Work out the finished part from the listing and answer in its coordinate system (mm). Round coordinates to 2 decimals unless told otherwise and drop trailing zeros. Loops run counter-clockwise (first coordinate to the right, second up) from the corner with the lowest first, then second, coordinate; pieces in that order, holes last.
Autodesk Inventor part; units mm, degrees
ref_plane "YZ Plane" through (0, 0, 0) normal (1, 0, 0) x (0, 1, 0)
ref_plane "XZ Plane" through (0, 0, 0) normal (0, 1, 0) x (-1, 0, 0)
ref_plane "XY Plane" through (0, 0, 0) normal (0, 0, 1) x (1, 0, 0)
sketch "Foam Scheme" plane through (0, 0, 0) normal (0, 1, 0) x (-1, 0, 0)
  line L0 (447, -94) -> (-447, -94)
  line L1 (-447, -94) -> (-447, 94)
  line L2 (-447, 94) -> (447, 94)
  line L3 (447, 94) -> (447, -94)
  circle A0 centre (425, -72) radius 9.5
  circle A1 centre (375, -72) radius 9.5
  circle A2 centre (325, -72) radius 9.5
  circle A3 centre (275, -72) radius 9.5
  circle A4 centre (225, -72) radius 9.5
  circle A5 centre (175, -72) radius 9.5
  circle A6 centre (125, -72) radius 9.5
  circle A7 centre (75, -72) radius 9.5
  circle A8 centre (25, -72) radius 9.5
  circle A9 centre (-25, -72) radius 9.5
  circle A10 centre (-75, -72) radius 9.5
  circle A11 centre (-125, -72) radius 9.5
  circle A12 centre (-175, -72) radius 9.5
  circle A13 centre (-225, -72) radius 9.5
  circle A14 centre (-275, -72) radius 9.5
  circle A15 centre (-325, -72) radius 9.5
  circle A16 centre (-375, -72) radius 9.5
  circle A17 centre (-425, -72) radius 9.5
  circle A18 centre (425, 72) radius 9.5
  circle A19 centre (375, 72) radius 9.5
  circle A20 centre (325, 72) radius 9.5
  circle A21 centre (275, 72) radius 9.5
  circle A22 centre (225, 72) radius 9.5
  circle A23 centre (175, 72) radius 9.5
  circle A24 centre (125, 72) radius 9.5
  circle A25 centre (75, 72) radius 9.5
  circle A26 centre (25, 72) radius 9.5
  circle A27 centre (-25, 72) radius 9.5
  circle A28 centre (-75, 72) radius 9.5
  circle A29 centre (-125, 72) radius 9.5
  circle A30 centre (-175, 72) radius 9.5
  circle A31 centre (-225, 72) radius 9.5
  circle A32 centre (-275, 72) radius 9.5
  circle A33 centre (-325, 72) radius 9.5
  circle A34 centre (-375, 72) radius 9.5
  circle A35 centre (-425, 72) radius 9.5
  point P0 (0, 0)
  dimension "d0" = 894
  dimension "d1" = 447
  dimension "d2" = 188
  dimension "d3" = 94
  dimension "d4" = 19
  dimension "d5" = 22
  dimension "d6" = 22
  dimension "d9" = 50
  dimension "d12" = 144
extrude "Foam Body" add sketch "Foam Scheme" along normal blind 1.5
properties part number "Foam NPS 6" material "Rubber, Silicone"
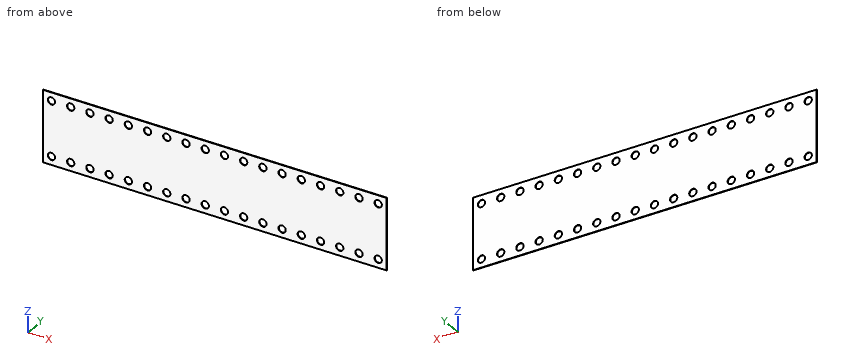
1. Given pin 1 (17 mm diameter, centred on x = 275, z = -72, fed in from +Y), flat-ended and moving along its own axis, determine where the tip first touches the part or whether it passes through.
Answer key:
pin 1: passes through
2. Find section B-B (z = 72). Give the number of separate pieces and of enclosed holes in the cut face, then the cut area to 3 significant figures.
Answer key:
separate pieces: 19
enclosed holes: 0
area: 828 mm2
3. Find section A-A (x = -325). Write down the section's boundary in (y, z), then the cut area to 3 significant figures.
Answer key:
outline: (0, -94) - (1.5, -94) - (1.5, -81.5) - (0, -81.5) - close; (0, -62.5) - (1.5, -62.5) - (1.5, 62.5) - (0, 62.5) - close; (0, 81.5) - (1.5, 81.5) - (1.5, 94) - (0, 94) - close
area: 225 mm2
4. Consider probe 1 along Z at (x, y) = (324.5, 0.55). Determine where the line is inside the solid, lowest interval first.
Answer key:
probe 1: z = -94 to -81.49, -62.51 to 62.51, 81.49 to 94
